Model file for the job. Use its own axes, mm. Give positions to 0.01 mm unless a question says otherwise; leave off trailing zeros. Write each loop counter-clockwise with the first axis right and the second up, starting at its lowest first coordinate (ties: lowest second). Pieces come first, ordered by that corner, then holes. Notation, with made-up numbers: (-23, 52) - (-14, 52) arc R14 cw to (-14, 65) - close; hole circle Ø6 at (16.5, -28). An arc over 180 degrees is marked (long way). One line per item, written item: value. Start each with the question number.
(1) Probe L1, parallel to Y at x = 73, z = -50.5; L2, parallel to Z at x = -81, y = -58.5; L3, parallel to X at y = -58.5, z = -52.5. List the from-to ranges inside material, lowest first.
(2) Cut at A-A, the plane x = -140.5. List the corners of the cut face in (y, z).
(3) Drop flat-ended pins along their axis: P1, Ø0.8, axis at y = -65.5, z = -29, coming from the +X side; P2, Ø3, axis at x = 205, z = -16, coming from the -Y side; P3, Ø0.8, axis at y = -65.5, z = -34, coming from the -X side. Give the stop position or say it passes through.
from build123d import *

# Parameters (mm, degrees)
F0_W     = 943
F0_H     = 58
F1_DEPTH = 65
F2_R     = 7
F3_W     = 60
F3_H     = 20
F4_DEPTH = 1


with BuildPart() as f1:
    # F0 (on Front) → F1 (new body)
    with BuildSketch(Plane.XZ):
        with Locations((0, -29)):
            Rectangle(F0_W, F0_H)
    extrude(amount=F1_DEPTH)

    # F2
    f2_edges = [f1.edges().sort_by_distance(p)[0] for p in [
        (0, -65, 0),
        (471.5, -32.5, 0),
        (471.5, -65, -29),
        (471.5, -32.5, -58),
        (0, -65, -58),
        (-471.5, -32.5, 0),
        (-471.5, -32.5, -58),
        (-471.5, -65, -29),
    ]]
    fillet(f2_edges, radius=F2_R)

    # F3 (on face) → F4 (join)
    with BuildSketch(Plane.XZ.offset(65)):
        with Locations((0, -29)):
            Rectangle(F3_W, F3_H)
    extrude(amount=F4_DEPTH)


solid = f1.part
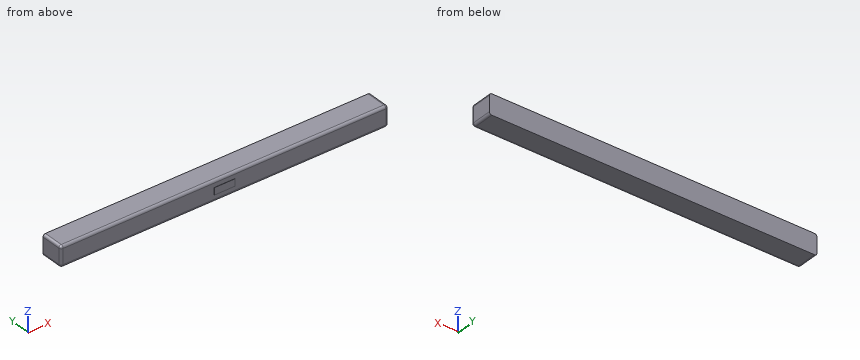
Answers follow:
1. L1: y = -65 to 0
1. L2: z = -57.98 to -0.02
1. L3: x = -471.32 to 471.32
2. outline: (-65, -51) arc R7 ccw to (-58, -58) - (0, -58) - (0, 0) - (-58, 0) arc R7 ccw to (-65, -7) - close
3. P1: stops at x = 30
3. P2: stops at y = -65
3. P3: stops at x = -30
